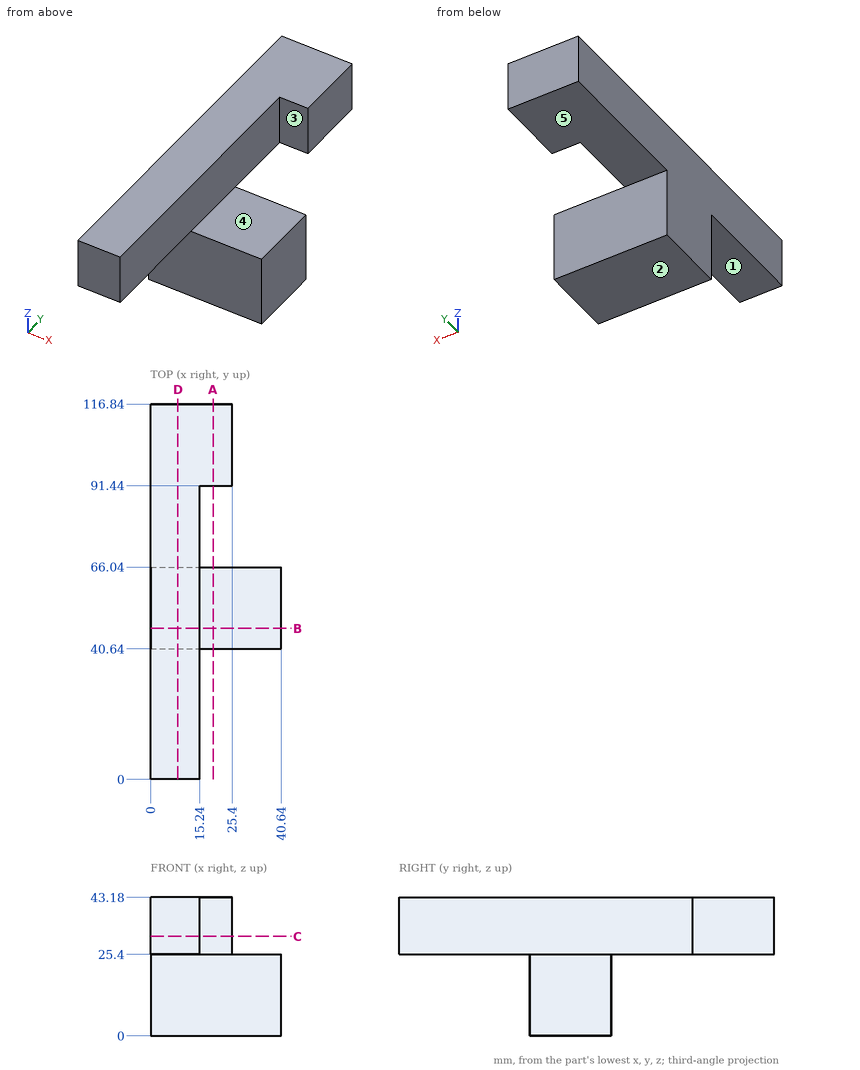
Check sheet for the drawn part. Datum: minimum x, y, z corner. Units: mm. A direction names the side the tool comes from. Coordinates: 2 decimals unless noted, no trailing zeros. Loops run counter-clockwise (first coordinate to the right, second up) from the corner with the lowest first, then second, coordinate; pieces in that order, holes last. Notation, with made-up numbers: (-36, 70.25) -> (-12, 70.25) arc R22 cw to (-12, 102.25) -> close; hole circle Ø5 at (21, 65). An arc over 180 degrees is marked (long way). Answer in a Markdown table with one row per item.
1. Sectioned sample at D-D, the plane x = 8.5. Record the boundary of the cut face in (y, z).
Check values:
| item | result |
|---|---|
| outline | (0, 25.4) -> (40.64, 25.4) -> (40.64, 0) -> (66.04, 0) -> (66.04, 25.4) -> (116.84, 25.4) -> (116.84, 43.18) -> (0, 43.18) -> close |
2. Access from +Z, -Z, +X, -X, +Y, -Y to the whole of each face (thin tool, end or side, straight path). Record for the marked faces 1, 2, 3, 4 and 5.
Check values:
| item | result |
|---|---|
| face 1 | -Z, +X, -X, -Y |
| face 2 | -Z, +X, -X, +Y, -Y |
| face 3 | +Z, -Z, +X, -Y |
| face 4 | +Z, +X, -Y |
| face 5 | -Z, +X, -X, +Y |
3. Sectioned sample at C-C, the plane z = 31. Record the boundary of the cut face in (x, y).
Check values:
| item | result |
|---|---|
| outline | (0, 0) -> (15.24, 0) -> (15.24, 91.44) -> (25.4, 91.44) -> (25.4, 116.84) -> (0, 116.84) -> close |
4. Sectioned sample at B-B, the plane y = 47. Record the boundary of the cut face in (x, z).
Check values:
| item | result |
|---|---|
| outline | (0, 0) -> (40.64, 0) -> (40.64, 25.4) -> (15.24, 25.4) -> (15.24, 43.18) -> (0, 43.18) -> close |
5. Material ranges on line 1 along Y through (x, z) = (33, 6); line 2 along Z through (x, y) = (20, 98.5); line 3 along X through (y, z) = (39, 26.5), recorded low to high. Write a range as [from, to].
Check values:
| item | result |
|---|---|
| line 1 | y = [40.64, 66.04] |
| line 2 | z = [25.4, 43.18] |
| line 3 | x = [0, 15.24] |
6. Go/stop test with flat-tipped pins: pin 1 (12 mm diameter, centred on x = 8.5, y = 26, fed in from -Z); pin 2 (7.5 mm diameter, centred on x = 25.5, y = 53, fed in from +Z); pin 3 (2 mm diameter, centred on x = 4.5, z = 14.5, fed in from +Y). Record where each tip stops, or that it passes through.
Check values:
| item | result |
|---|---|
| pin 1 | stops at z = 25.4 |
| pin 2 | stops at z = 25.4 |
| pin 3 | stops at y = 66.04 |
7. Sectioned sample at A-A, the plane x = 19.5. Record the boundary of the cut face in (y, z).
Check values:
| item | result |
|---|---|
| outline | (40.64, 0) -> (66.04, 0) -> (66.04, 25.4) -> (40.64, 25.4) -> close; (91.44, 25.4) -> (116.84, 25.4) -> (116.84, 43.18) -> (91.44, 43.18) -> close |
